```python
from build123d import *

# Parameters (mm, degrees)
SZKIC5_R                                             = 1.5
DODANIE_WYCI_GNI_CIE2_DEPTH                          = 24
POG_BIENIE_WALCOWE_POD_M3_WKR_T_DO_CZ_CI_D           = 3.4
POG_BIENIE_WALCOWE_POD_M3_WKR_T_DO_CZ_CI_CBORE_D     = 7
POG_BIENIE_WALCOWE_POD_M3_WKR_T_DO_CZ_CI_CBORE_DEPTH = 2.4
SZKIC14_W                                            = 16
SZKIC14_H                                            = 17
WYTNIJ_WYCI_GNI_CIE1_DEPTH                           = 9
WYTNIJ_WYCI_GNI_CIE1_DEPTH_BACK                      = 24
WYTNIJ_WYCI_GNI_CIE2_DEPTH                           = 8


with BuildPart() as part:
    # Szkic5 → Dodanie-wyciągnięcie2 (new body)
    with BuildSketch(Plane(origin=(0, 0, 0), x_dir=(0, 0, -1), z_dir=(1, 0, 0))):
        with BuildLine():
            Line((-12.908163265, 21.275510204), (-12.908163265, -3.724489796))
            ThreePointArc((-12.908163265, -3.724489796), (-6.408163265, -10.224489796), (0.091836735, -3.724489796))
            ThreePointArc((0.091836735, -3.724489796), (6.591813696, 5.834724726), (1.9156302, 16.406460189))
            ThreePointArc((1.9156302, 16.406460189), (-5.106681022, 20.027075938), (-12.908163265, 21.275510204))
        make_face()
        with Locations((-6.408163265, -3.724489796)):
            Circle(SZKIC5_R, mode=Mode.SUBTRACT)
    extrude(amount=DODANIE_WYCI_GNI_CIE2_DEPTH)

    # Pogłębienie walcowe pod M3 wkręt do części metalowych z łbem stożkowym ściętym1 (through all)
    with Locations(Plane(origin=(24, 0, 0), x_dir=(0, 0, -1), z_dir=(1, 0, 0))):
        with Locations((-0.443639472, 11.715274148)):
            CounterBoreHole(POG_BIENIE_WALCOWE_POD_M3_WKR_T_DO_CZ_CI_D / 2, POG_BIENIE_WALCOWE_POD_M3_WKR_T_DO_CZ_CI_CBORE_D / 2, POG_BIENIE_WALCOWE_POD_M3_WKR_T_DO_CZ_CI_CBORE_DEPTH)

    # Szkic14 → Wytnij-wyciągnięcie1 (cut, two sides)
    with BuildSketch(Plane.XY) as wytnij_wyci_gni_cie1_sk:
        with Locations((12, 10.775510204)):
            Rectangle(SZKIC14_W, SZKIC14_H)
    extrude(amount=WYTNIJ_WYCI_GNI_CIE1_DEPTH, mode=Mode.SUBTRACT)
    extrude(wytnij_wyci_gni_cie1_sk.sketch, amount=-WYTNIJ_WYCI_GNI_CIE1_DEPTH_BACK, mode=Mode.SUBTRACT)

    # Szkic18 → Wytnij-wyciągnięcie2 (cut)
    with BuildSketch(Plane.ZY):
        Polygon((1.412173102, 7.834302284), (4.288926512, 10.613562944), (3.320392883, 14.494534808), (-0.524894158, 15.596246012), (-3.401647568, 12.816985352), (-2.433113939, 8.936013488), align=None)
    extrude(amount=-WYTNIJ_WYCI_GNI_CIE2_DEPTH, mode=Mode.SUBTRACT)


solid = part.part
```
Input: part model. Units: mm. Frame: model coordinates. A direction names the side the tool comes from. Coordinates: 2 decimals unless noted, no trailing zeros. Loops run counter-clockwise (first coordinate to the right, second up) from the corner with the lowest first, then second, coordinate; pieces in that order, holes last. Notation, with made-up numbers: (66.25, 42) -> (79.25, 42) arc R20 ccw to (79.25, 52) -> close; hole circle Ø10 at (79, 32). An arc over 180 degrees is marked (long way). Use a Markdown table: item, result.
1) Cut plane D-D (z = -5.25). Return the cut outline in (x, y), then the cut area to 3 significant figures.
Results found:
| item | result |
|---|---|
| outline | (0, 1.33) -> (24, 1.33) -> (24, 12.49) -> (20, 12.49) -> (20, 2.28) -> (4, 2.28) -> (4, 12.49) -> (0, 12.49) -> close |
| area | 105 mm2 |
2) Pull-direction query (Y, two-part tool) for faces 1 (the cylindrical face through (11.83, 0.63, -4.85)), 2 (the flat face through (24, 6, 5)), 3 (the cylindrical face through (20.789, 10.056, 0.075)); classes: released by +Y, released by -Y, zero draft, split by the parting line, or undercut.
Results found:
| item | result |
|---|---|
| face 1 | split by the parting line |
| face 2 | zero draft |
| face 3 | undercut |
3) Cut plane C-C (y = 5). Return the cut outline in (x, z), then the cut area to 3 significant figures.
Results found:
| item | result |
|---|---|
| outline | (0, -6.49) -> (4, -6.49) -> (4, 9) -> (20, 9) -> (20, -6.49) -> (24, -6.49) -> (24, 12.91) -> (0, 12.91) -> close |
| area | 218 mm2 |
4) Access query for faces 4 (the cylindrical face through (22.817, 15.185, 0.899)), 5 (the cylindrical face through (11.832, -10.223, 6.551)), 6 (the flat face through (1.97, 15.04, 1.42)), 7 (the cylindrical face through (11.83, 20.49, 6.69)), 8 (the flat face through (12, 2.276, 2)). Directions: +Z, -Z, +X, -X, +Y, -Y. A direction counts if a zero-diameter tool reaches every point of the face in a straight line with its end or side. Return the directions, or none.
Results found:
| item | result |
|---|---|
| face 4 | +X |
| face 5 | +X, -X, -Y |
| face 6 | -X |
| face 7 | -Z, +X, -X, +Y |
| face 8 | -Z |
5) Cut plane A-A (x = 6). Return the cut outline in (y, z), then the cut area to 3 significant figures.
Results found:
| item | result |
|---|---|
| outline | (-3.72, -0.09) arc R11.91 ccw to (2.28, -5.7) -> (2.28, 9) -> (19.28, 9) -> (19.28, 3.11) arc R25 ccw to (21.28, 12.91) -> (-3.72, 12.91) arc R6.5 ccw to start; hole circle Ø3 at (-3.72, 6.41) |
| area | 238 mm2 |
6) Contact query for flat-ended pins moving along their axis: pin 1 (1 mm diameter, centred on y = 14.5, z = 9.5, fed in from -X); pin 2 (1.5 mm diameter, centred on x = 5, z = 2, fed in from +Y); pin 3 (2.5 mm diameter, centred on y = 11.72, z = 0.44, fed in from -X); pin 4 (5.5 mm diameter, centred on y = 11.72, z = 0.44, fed in from -X). Output: stop coordinate, or through.
Results found:
| item | result |
|---|---|
| pin 1 | stops at x = 0 |
| pin 2 | stops at y = 2.28 |
| pin 3 | passes through |
| pin 4 | stops at x = 20 |
7) Material intervals for line 1 along X through (y, z) = (7.5, -3.25); line 2 along Z through (x, y) = (22.75, 7); line 3 along Z through (x, y) = (8.75, 6), sorted ascending. Write a range as from..to.
Results found:
| item | result |
|---|---|
| line 1 | x = 0..4, 20..24 |
| line 2 | z = -6.64..12.91 |
| line 3 | z = 9..12.91 |
8) Cut plane B-B (y = 14). Return the cut outline in (x, z), then the cut area to 3 significant figures.
Results found:
| item | result |
|---|---|
| outline | (0, -4.3) -> (4, -4.3) -> (4, -2.18) -> (0, -2.18) -> close; (0, 3.44) -> (4, 3.44) -> (4, 9) -> (20, 9) -> (20, -4.3) -> (24, -4.3) -> (24, -2.21) -> (21.6, -2.21) -> (21.6, 3.1) -> (24, 3.1) -> (24, 12.91) -> (0, 12.91) -> close |
| area | 165 mm2 |
